Verification items for this drawing (mm, ordinates from the low corner). A direction names the side the tool comes from. Give positions to 0.01 mm unless a question says otherwise; leave off trailing zeros. Order: outer loops, then holes, each group sorted by start corner. A loop starts at its lowest first (then second) coordinate and runs counter-clockwise, first axis right, second up.
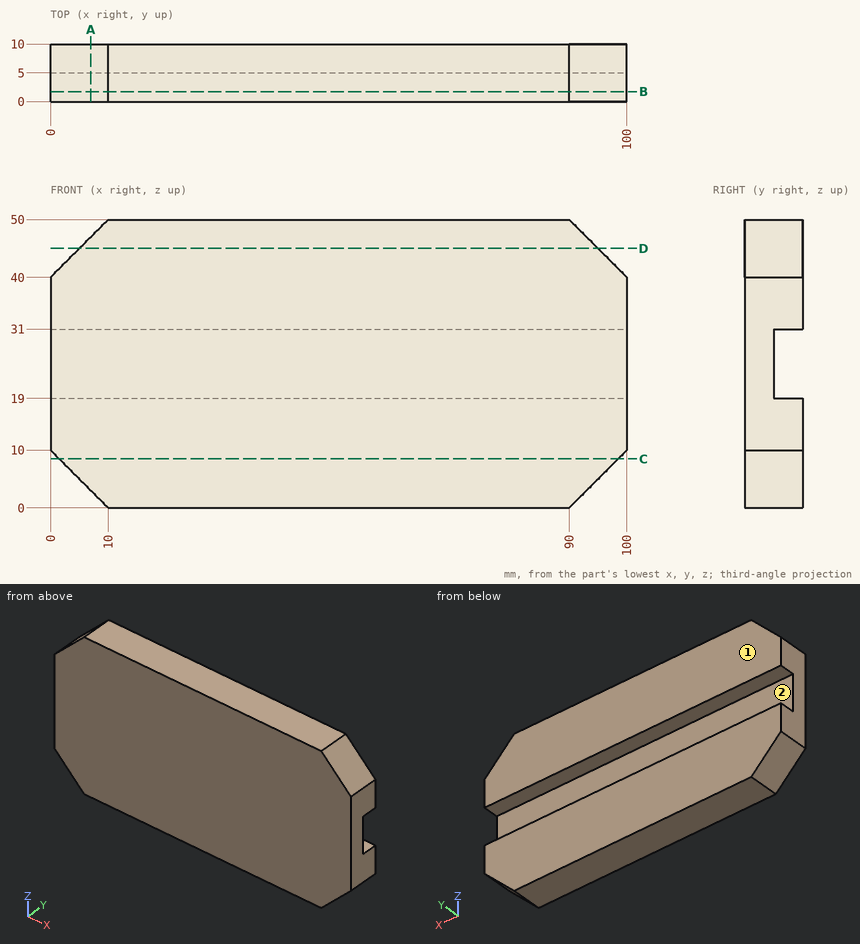
Q1. Cross-section at B-B, the plane y = 1.75. Record the boundary of the cut face in (x, z).
Q2. Cross-section at A-A, the plane x = 7. Record the boundary of the cut face in (y, z), and give its area (3 significant figures).
Q3. Thickness scan on L1, parallel to Z at x = 58, y = 7.25; L2, parallel to Y at x = 22, z = 22; L3, parallel to Z at x = 5.5, y = 1.5. Record the ranges inside material, lowest first.
Q4. Cross-section at C-C, the plane z = 8.5. Record the boundary of the cut face in (x, y).
Q5. Access from +Z, -Z, +X, -X, +Y, -Y to the whole of each face (thin tool, end or side, straight path). Record for the marked faces 1 and 2.
Q6. Cross-section at D-D, the plane z = 45. Record the boundary of the cut face in (x, y).
Answers follow:
1. outline: (0, 10) - (10, 0) - (90, 0) - (100, 10) - (100, 40) - (90, 50) - (10, 50) - (0, 40) - close
2. outline: (0, 3) - (10, 3) - (10, 19) - (5, 19) - (5, 31) - (10, 31) - (10, 47) - (0, 47) - close
2. area: 380 mm2
3. L1: z = 0 to 19, 31 to 50
3. L2: y = 0 to 5
3. L3: z = 4.5 to 45.5
4. outline: (1.5, 0) - (98.5, 0) - (98.5, 10) - (1.5, 10) - close
5. face 1: +Z, -Z, +X, -X, +Y
5. face 2: +X, -X, +Y
6. outline: (5, 0) - (95, 0) - (95, 10) - (5, 10) - close
